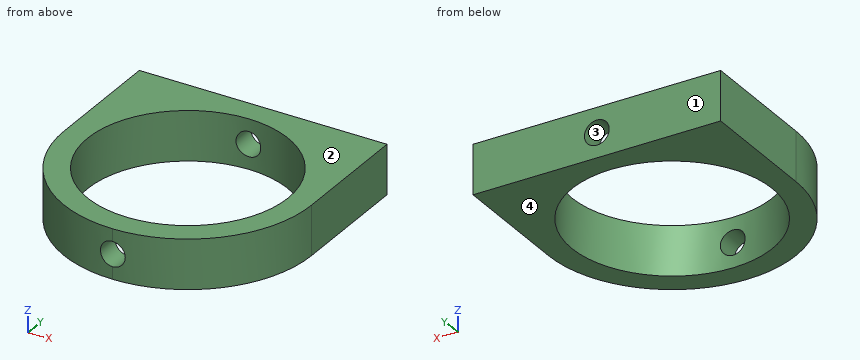
```python
from build123d import *

# Parameters (mm, degrees)
SKETCH1_R           = 8.1
BOSS_EXTRUDE1_DEPTH = 4
SKETCH3_R           = 1
CUT_EXTRUDE1_DEPTH  = 20


with BuildPart() as part:
    # Sketch1 → Boss-Extrude1 (new body)
    with BuildSketch(Plane.XY):
        with BuildLine():
            ThreePointArc((-10, 0), (-7.071067812, -7.071067812), (0, -10))
            ThreePointArc((0, -10), (7.071067812, -7.071067812), (10, 0))
            Line((10, 0), (10, 10))
            Line((10, 10), (-10, 10))
            Line((-10, 10), (-10, 0))
        make_face()
        Circle(SKETCH1_R, mode=Mode.SUBTRACT)
    extrude(amount=BOSS_EXTRUDE1_DEPTH)

    # Sketch3 → Cut-Extrude1 (cut)
    with BuildSketch(Plane(origin=(0, 10, 0), x_dir=(1, 0, 0), z_dir=(0, 1, 0))):
        with Locations(Location((0, -2, 0), (0, 0, 270))):
            Circle(SKETCH3_R)
    extrude(amount=-CUT_EXTRUDE1_DEPTH, mode=Mode.SUBTRACT)


solid = part.part
```
Input: part model. Units: mm. Frame: model coordinates. Face numbers are marked on the shaded views. Coordinates: 2 decimals unless noted, no trailing zeros. Write each loop counter-clockwise with the first axis right and the second up, starting at its lowest first coordinate (ties: lowest second). Pieces come first, ordered by that corner, then holes.
1) Section B-B on x = -6. Output: boundary loops of the cut face in (y, z), and give its area (3 significant figures).
2) Material intervals for line 1 along Y through (x, z) = (-0.25, 3.35); line 2 along Z through (x, y) = (0, -8.55); line 3 along X through (y, z) = (-1, 2.1), sorted ascending.
3) Section C-C on y = 6.5. Output: boundary loops of the cut face in (x, z), and give its area (3 significant figures).
4) Mould query, pull axis Z, two halves, no side actions, for the marked faces 1, 2, 3 and 4. Classes: pulls with the +Z half, pulls with the -Z half, needs draft (parallel to the pull), parting line crosses it, or undercut.
5) Pin query (flat end, axial travel): pin 1 Ø1.2 at (x, z) = (0, 2) entering from -Y. Return the tip coordinate at first contact, or that it passes through.
6) Section A-A on z = 1.8. Output: boundary loops of the cut face in (x, y), and give its area (3 significant figures).
Check result:
1. outline: (-8, 0) - (-5.44, 0) - (-5.44, 4) - (-8, 4) - close; (5.44, 0) - (10, 0) - (10, 4) - (5.44, 4) - close
1. area: 28.5 mm2
2. line 1: y = -10 to -8.1, 8.1 to 10
2. line 2: z = 0 to 1, 3 to 4
2. line 3: x = -9.95 to -8.04, 8.04 to 9.95
3. outline: (-10, 0) - (-4.83, 0) - (-4.83, 4) - (-10, 4) - close; (4.83, 0) - (10, 0) - (10, 4) - (4.83, 4) - close
3. area: 41.3 mm2
4. face 1: needs draft
4. face 2: pulls with the +Z half
4. face 3: undercut
4. face 4: pulls with the -Z half
5. pin 1: passes through
6. outline: (-10, 0) arc R10 ccw to (-0.98, -9.95) - (-0.98, -8.04) arc R8.1 cw to (-0.98, 8.04) - (-0.98, 10) - (-10, 10) - close; (0.98, -9.95) arc R10 ccw to (10, 0) - (10, 10) - (0.98, 10) - (0.98, 8.04) arc R8.1 cw to (0.98, -8.04) - close
6. area: 143 mm2
